from build123d import *

# Parameters (mm, degrees)
SKETCH1_R           = 4.7625
BOSS_EXTRUDE2_DEPTH = 25.4
SKETCH4_R           = 2.413
BOSS_EXTRUDE3_DEPTH = 4.7625
SKETCH5_R           = 2.5527
CUT_EXTRUDE2_DEPTH  = 19.05


with BuildPart() as part:
    # Sketch1 → Boss-Extrude2 (new body)
    with BuildSketch(Plane.XY):
        Circle(SKETCH1_R)
    extrude(amount=BOSS_EXTRUDE2_DEPTH)

    # Sketch4 → Boss-Extrude3 (add)
    with BuildSketch(Plane.XY.offset(25.4)):
        with Locations((0.635, 0)):
            Circle(SKETCH4_R)
    extrude(amount=BOSS_EXTRUDE3_DEPTH)

    # Sketch5 → Cut-Extrude2 (cut)
    with BuildSketch(Plane(origin=(0, 0, 0), x_dir=(-1, 0, 0), z_dir=(0, 0, -1))):
        Circle(SKETCH5_R)
    extrude(amount=-CUT_EXTRUDE2_DEPTH, mode=Mode.SUBTRACT)


solid = part.part
Verification items for the finished model (mm, model axes). A direction names the side the tool comes from. Coordinates: 2 decimals unless noted, no trailing zeros. Write each loop counter-clockwise with the first axis right and the second up, starting at its lowest first coordinate (ties: lowest second). Pieces come first, ordered by that corner, then holes. Notation, with made-up numbers: M 81,30 L 139,30 A25 ccw 139,51 Z; hole C -25,3.5 d7. An arc over 180 degrees is marked long. Use a Markdown table: item, result.
Q1. Sectioned sample at A-A, the plane y = 0. Record the boundary of the cut face in (x, z), plus the area to 3 significant figures.
Reply:
| item | result |
|---|---|
| outline | M -4.76,0 L -2.55,0 L -2.55,19.05 L 2.55,19.05 L 2.55,0 L 4.76,0 L 4.76,25.4 L 3.05,25.4 L 3.05,30.16 L -1.78,30.16 L -1.78,25.4 L -4.76,25.4 Z |
| area | 168 mm² |
Q2. Go/stop test with flat-tipped pins: P1, Ø1, axis at y = -4, z = 9, coming from the -X side; P2, Ø1.5, axis at x = 1.5, z = 17.5, coming from the -Y side. Record where each tip stops, or that it passes through.
Reply:
| item | result |
|---|---|
| P1 | stops at x = -3.23 |
| P2 | stops at y = -4.7 |
Q3. Thickness scan on line 1 (Y direction, x = 0, z = 14.5); line 2 (Z direction, x = -1, y = 0.75); line 3 (Z direction, x = 2, y = -3.75). Record the ranges inside material, lowest first.
Reply:
| item | result |
|---|---|
| line 1 | y = -4.76 to -2.55, 2.55 to 4.76 |
| line 2 | z = 19.05 to 30.16 |
| line 3 | z = 0 to 25.4 |
Q4. Sectioned sample at D-D, the plane z = 4.5. Record the boundary of the cut face in (x, y) (1 decimal).
Reply:
| item | result |
|---|---|
| outline | C 0,0 d9.5; hole C 0,0 d5.1 |
Q5. Sectioned sample at C-C, the plane x = 0. Record the boundary of the cut face in (y, z), plus the area to 3 significant figures.
Reply:
| item | result |
|---|---|
| outline | M -4.76,0 L -2.55,0 L -2.55,19.05 L 2.55,19.05 L 2.55,0 L 4.76,0 L 4.76,25.4 L 2.33,25.4 L 2.33,30.16 L -2.33,30.16 L -2.33,25.4 L -4.76,25.4 Z |
| area | 167 mm² |
Q6. Set-up check for faces 1 (the face through (-1.28, -1.47, 27.75)), 2 (the face through (1, 0, 30.162)): record each of +Z, -Z, +X, -X, +Y, -Y from which the full face is reachable in a straight line by a thin tool's end or side.
Reply:
| item | result |
|---|---|
| face 1 | +Z |
| face 2 | +Z, +X, -X, +Y, -Y |
Q7. Draft check along X on faces 3 (the face through (0, 0, 19.05)), 4 (the face through (2, -2, 0)), 5 (the face through (-3.78, -2.9, 12.52)), 6 (the face through (-2.435, 0.767, 9.392)). Enter one of: +X half, -X half, draft (parallel to the pull), parting line (faces both ways), or undercut.
Reply:
| item | result |
|---|---|
| face 3 | undercut |
| face 4 | draft |
| face 5 | parting line |
| face 6 | undercut |
Q8. Sectioned sample at B-B, the plane z = 27.5. Record the boundary of the cut face in (x, y) (3 decimals).
Reply:
| item | result |
|---|---|
| outline | C 0.635,0 d4.826 |
